Source: CAD feature listing. Evaluate the final solid. Frame: model axes, mm. A direction names the side the tool comes from. Give positions to 0.01 mm unless a question says otherwise; leave off trailing zeros. Order: outer loops, then holes, each group sorted by start corner. A loop starts at its lowest first (then second) coordinate and runs counter-clockwise, first axis right, second up. Notation, with made-up numbers: (15.5, 61.5) - (62.5, 61.5) arc R20 cw to (62.5, 72.5) - close; hole circle Ø1 at (48, 73). An arc over 180 degrees is marked (long way). Answer as CSV lines item,"result".
```python
from build123d import *

# Parameters (mm, degrees)
BOSS_EXTRUDE1_DEPTH = 35
SKETCH3_W           = 5.25
SKETCH3_H           = 5.25
CUT_EXTRUDE2_DEPTH  = 10.2
CUT_EXTRUDE3_START  = -35
SKETCH3_2_W         = 5.25
SKETCH3_2_H         = 5.25
CUT_EXTRUDE3_DEPTH  = 10


with BuildPart() as part:
    # Sketch1 → Boss-Extrude1 (new body)
    with BuildSketch(Plane(origin=(0, 0, 0), x_dir=(0, 0, -1), z_dir=(1, 0, 0))):
        with BuildLine():
            Line((-1, 11.732050808), (0, 10))
            Line((0, 10), (1, 11.732050808))
            ThreePointArc((1, 11.732050808), (1.026223309, 11.729786097), (1.05244149, 11.727462772))
            Line((1.05244149, 11.727462772), (1.736481777, 9.84807753))
            Line((1.736481777, 9.84807753), (3.022056996, 11.380166416))
            ThreePointArc((3.022056996, 11.380166416), (3.047488651, 11.373382482), (3.072905078, 11.366541714))
            Line((3.072905078, 11.366541714), (3.420201433, 9.396926208))
            Line((3.420201433, 9.396926208), (4.952290319, 10.682501427))
            ThreePointArc((4.952290319, 10.682501427), (4.976157593, 10.671404395), (5, 10.660254038))
            Line((5, 10.660254038), (5, 8.660254038))
            Line((5, 8.660254038), (6.732050808, 9.660254038))
            ThreePointArc((6.732050808, 9.660254038), (6.753628504, 9.645181086), (6.775172452, 9.630059937))
            Line((6.775172452, 9.630059937), (6.427876097, 7.660444431))
            Line((6.427876097, 7.660444431), (8.307261338, 8.344484718))
            ThreePointArc((8.307261338, 8.344484718), (8.32589383, 8.32589383), (8.344484718, 8.307261338))
            Line((8.344484718, 8.307261338), (7.660444431, 6.427876097))
            Line((7.660444431, 6.427876097), (9.630059937, 6.775172452))
            ThreePointArc((9.630059937, 6.775172452), (9.645181086, 6.753628504), (9.660254038, 6.732050808))
            Line((9.660254038, 6.732050808), (8.660254038, 5))
            Line((8.660254038, 5), (10.660254038, 5))
            ThreePointArc((10.660254038, 5), (10.671404395, 4.976157593), (10.682501427, 4.952290319))
            Line((10.682501427, 4.952290319), (9.396926208, 3.420201433))
            Line((9.396926208, 3.420201433), (11.366541714, 3.072905078))
            ThreePointArc((11.366541714, 3.072905078), (11.373382482, 3.047488651), (11.380166416, 3.022056996))
            Line((11.380166416, 3.022056996), (9.84807753, 1.736481777))
            Line((9.84807753, 1.736481777), (11.727462772, 1.05244149))
            ThreePointArc((11.727462772, 1.05244149), (11.729786097, 1.026223309), (11.732050808, 1))
            Line((11.732050808, 1), (10, 0))
            Line((10, 0), (11.732050808, -1))
            ThreePointArc((11.732050808, -1), (11.729786097, -1.026223309), (11.727462772, -1.05244149))
            Line((11.727462772, -1.05244149), (9.84807753, -1.736481777))
            Line((9.84807753, -1.736481777), (11.380166416, -3.022056996))
            ThreePointArc((11.380166416, -3.022056996), (11.373382482, -3.047488651), (11.366541714, -3.072905078))
            Line((11.366541714, -3.072905078), (9.396926208, -3.420201433))
            Line((9.396926208, -3.420201433), (10.682501427, -4.952290319))
            ThreePointArc((10.682501427, -4.952290319), (10.671404395, -4.976157593), (10.660254038, -5))
            Line((10.660254038, -5), (8.660254038, -5))
            Line((8.660254038, -5), (9.660254038, -6.732050808))
            ThreePointArc((9.660254038, -6.732050808), (9.645181086, -6.753628504), (9.630059937, -6.775172452))
            Line((9.630059937, -6.775172452), (7.660444431, -6.427876097))
            Line((7.660444431, -6.427876097), (8.344484718, -8.307261338))
            ThreePointArc((8.344484718, -8.307261338), (8.32589383, -8.32589383), (8.307261338, -8.344484718))
            Line((8.307261338, -8.344484718), (6.427876097, -7.660444431))
            Line((6.427876097, -7.660444431), (6.775172452, -9.630059937))
            ThreePointArc((6.775172452, -9.630059937), (6.753628504, -9.645181086), (6.732050808, -9.660254038))
            Line((6.732050808, -9.660254038), (5, -8.660254038))
            Line((5, -8.660254038), (5, -10.660254038))
            ThreePointArc((5, -10.660254038), (4.976157593, -10.671404395), (4.952290319, -10.682501427))
            Line((4.952290319, -10.682501427), (3.420201433, -9.396926208))
            Line((3.420201433, -9.396926208), (3.072905078, -11.366541714))
            ThreePointArc((3.072905078, -11.366541714), (3.047488651, -11.373382482), (3.022056996, -11.380166416))
            Line((3.022056996, -11.380166416), (1.736481777, -9.84807753))
            Line((1.736481777, -9.84807753), (1.05244149, -11.727462772))
            ThreePointArc((1.05244149, -11.727462772), (1.026223309, -11.729786097), (1, -11.732050808))
            Line((1, -11.732050808), (0, -10))
            Line((0, -10), (-1, -11.732050808))
            ThreePointArc((-1, -11.732050808), (-1.026223309, -11.729786097), (-1.05244149, -11.727462772))
            Line((-1.05244149, -11.727462772), (-1.736481777, -9.84807753))
            Line((-1.736481777, -9.84807753), (-3.022056996, -11.380166416))
            ThreePointArc((-3.022056996, -11.380166416), (-3.047488651, -11.373382482), (-3.072905078, -11.366541714))
            Line((-3.072905078, -11.366541714), (-3.420201433, -9.396926208))
            Line((-3.420201433, -9.396926208), (-4.952290319, -10.682501427))
            ThreePointArc((-4.952290319, -10.682501427), (-4.976157593, -10.671404395), (-5, -10.660254038))
            Line((-5, -10.660254038), (-5, -8.660254038))
            Line((-5, -8.660254038), (-6.732050808, -9.660254038))
            ThreePointArc((-6.732050808, -9.660254038), (-6.753628504, -9.645181086), (-6.775172452, -9.630059937))
            Line((-6.775172452, -9.630059937), (-6.427876097, -7.660444431))
            Line((-6.427876097, -7.660444431), (-8.307261338, -8.344484718))
            ThreePointArc((-8.307261338, -8.344484718), (-8.32589383, -8.32589383), (-8.344484718, -8.307261338))
            Line((-8.344484718, -8.307261338), (-7.660444431, -6.427876097))
            Line((-7.660444431, -6.427876097), (-9.630059937, -6.775172452))
            ThreePointArc((-9.630059937, -6.775172452), (-9.645181086, -6.753628504), (-9.660254038, -6.732050808))
            Line((-9.660254038, -6.732050808), (-8.660254038, -5))
            Line((-8.660254038, -5), (-10.660254038, -5))
            ThreePointArc((-10.660254038, -5), (-10.671404395, -4.976157593), (-10.682501427, -4.952290319))
            Line((-10.682501427, -4.952290319), (-9.396926208, -3.420201433))
            Line((-9.396926208, -3.420201433), (-11.366541714, -3.072905078))
            ThreePointArc((-11.366541714, -3.072905078), (-11.373382482, -3.047488651), (-11.380166416, -3.022056996))
            Line((-11.380166416, -3.022056996), (-9.84807753, -1.736481777))
            Line((-9.84807753, -1.736481777), (-11.727462772, -1.05244149))
            ThreePointArc((-11.727462772, -1.05244149), (-11.729786097, -1.026223309), (-11.732050808, -1))
            Line((-11.732050808, -1), (-10, 0))
            Line((-10, 0), (-11.732050808, 1))
            ThreePointArc((-11.732050808, 1), (-11.729786097, 1.026223309), (-11.727462772, 1.05244149))
            Line((-11.727462772, 1.05244149), (-9.84807753, 1.736481777))
            Line((-9.84807753, 1.736481777), (-11.380166416, 3.022056996))
            ThreePointArc((-11.380166416, 3.022056996), (-11.373382482, 3.047488651), (-11.366541714, 3.072905078))
            Line((-11.366541714, 3.072905078), (-9.396926208, 3.420201433))
            Line((-9.396926208, 3.420201433), (-10.682501427, 4.952290319))
            ThreePointArc((-10.682501427, 4.952290319), (-10.671404395, 4.976157593), (-10.660254038, 5))
            Line((-10.660254038, 5), (-8.660254038, 5))
            Line((-8.660254038, 5), (-9.660254038, 6.732050808))
            ThreePointArc((-9.660254038, 6.732050808), (-9.645181086, 6.753628504), (-9.630059937, 6.775172452))
            Line((-9.630059937, 6.775172452), (-7.660444431, 6.427876097))
            Line((-7.660444431, 6.427876097), (-8.344484718, 8.307261338))
            ThreePointArc((-8.344484718, 8.307261338), (-8.32589383, 8.32589383), (-8.307261338, 8.344484718))
            Line((-8.307261338, 8.344484718), (-6.427876097, 7.660444431))
            Line((-6.427876097, 7.660444431), (-6.775172452, 9.630059937))
            ThreePointArc((-6.775172452, 9.630059937), (-6.753628504, 9.645181086), (-6.732050808, 9.660254038))
            Line((-6.732050808, 9.660254038), (-5, 8.660254038))
            Line((-5, 8.660254038), (-5, 10.660254038))
            ThreePointArc((-5, 10.660254038), (-4.976157593, 10.671404395), (-4.952290319, 10.682501427))
            Line((-4.952290319, 10.682501427), (-3.420201433, 9.396926208))
            Line((-3.420201433, 9.396926208), (-3.072905078, 11.366541714))
            ThreePointArc((-3.072905078, 11.366541714), (-3.047488651, 11.373382482), (-3.022056996, 11.380166416))
            Line((-3.022056996, 11.380166416), (-1.736481777, 9.84807753))
            Line((-1.736481777, 9.84807753), (-1.05244149, 11.727462772))
            ThreePointArc((-1.05244149, 11.727462772), (-1.026223309, 11.729786097), (-1, 11.732050808))
        make_face()
    extrude(amount=BOSS_EXTRUDE1_DEPTH)

    # Sketch3 → Cut-Extrude2 (cut)
    with BuildSketch(Plane(origin=(35, 0, 0), x_dir=(0, 0, -1), z_dir=(1, 0, 0))):
        with Locations((0.125, -0.125)):
            Rectangle(SKETCH3_W, SKETCH3_H)
    extrude(amount=-CUT_EXTRUDE2_DEPTH, mode=Mode.SUBTRACT)

    # Sketch3<2> → Cut-Extrude3 (cut)
    with BuildSketch(Plane(origin=(35, 0, 0), x_dir=(0, 0, -1), z_dir=(1, 0, 0)).offset(CUT_EXTRUDE3_START)):
        with Locations((0.125, -0.125)):
            Rectangle(SKETCH3_2_W, SKETCH3_2_H)
    extrude(amount=CUT_EXTRUDE3_DEPTH, mode=Mode.SUBTRACT)


solid = part.part
```
(1) Mould query, pull axis Z, two halves, no side actions, for faces 4 (the flat face through (17.26, -9.17, -5.88)), 5 (the flat face through (17.26, 5.88, -9.17)), 6 (the flat face through (17, -5, -10)), 7 (the flat face through (17.26, -10.8, 1.39)). Classes: released by +Z, released by -Z, zero draft, split by the parting line, or undercut.
Completed:
face 4,"undercut"
face 5,"released by -Z"
face 6,"zero draft"
face 7,"undercut"
(2) Ray query, line 1 (Y direction, x = 23, z = 9); line 2 (Y direction, x = 11.5, z = -10.5). Return the intervals inside material, ascending. Write a range as from..to.
Completed:
line 1,"-6.66..-5.59, -5..5, 5.59..6.66"
line 2,"-5..-4.73, -3.23..-2.28, -1.5..-0.29, 0.29..1.5, 2.28..3.23, 4.73..5"
(3) Access query for faces 1 (the flat face through (17.26, -8.63, -6.6)), 2 (the flat face through (17.26, 10.8, -1.39)), 3 (the flat face through (10, 0, 0)). Directions: +Z, -Z, +X, -X, +Y, -Y. A direction counts if a zero-diameter tool reaches every point of the face in a straight line with its end or side. Return the directions, or none.
Completed:
face 1,"+X, -X"
face 2,"+X, -X, +Y"
face 3,"-X"
(4) Cut plane B-B (y = 4.25). Return loops of the section in (x, z), then the cut area to 3 significant figures.
Completed:
outline,"(0, -10.09) - (35, -10.09) - (35, 10.09) - (0, 10.09) - close"
area,"707 mm²"
(5) Cut plane A-A (z = 0.5). Return loops of the section in (x, y).
Completed:
outline,"(0, -10.87) - (35, -10.87) - (35, -2.75) - (24.8, -2.75) - (24.8, 2.5) - (35, 2.5) - (35, 10.87) - (0, 10.87) - (0, 2.5) - (10, 2.5) - (10, -2.75) - (0, -2.75) - close"
(6) Contact query for flat-ended pins moving along their axis: pin 1 (2.5 mm diameter, centred on x = 31.5, y = -0.5, fed in from +Z); pin 2 (6 mm diameter, centred on x = 9.5, z = 5, fed in from +Y); pin 3 (1 mm diameter, centred on x = 20, y = -10, fed in from +Z); pin 4 (1.6 mm diameter, centred on y = 1, z = 0.5, fed in from -X). Output: stop coordinate, or through.
Completed:
pin 1,"z = 11.73"
pin 2,"y = 11.38"
pin 3,"z = 6.78"
pin 4,"x = 10"
